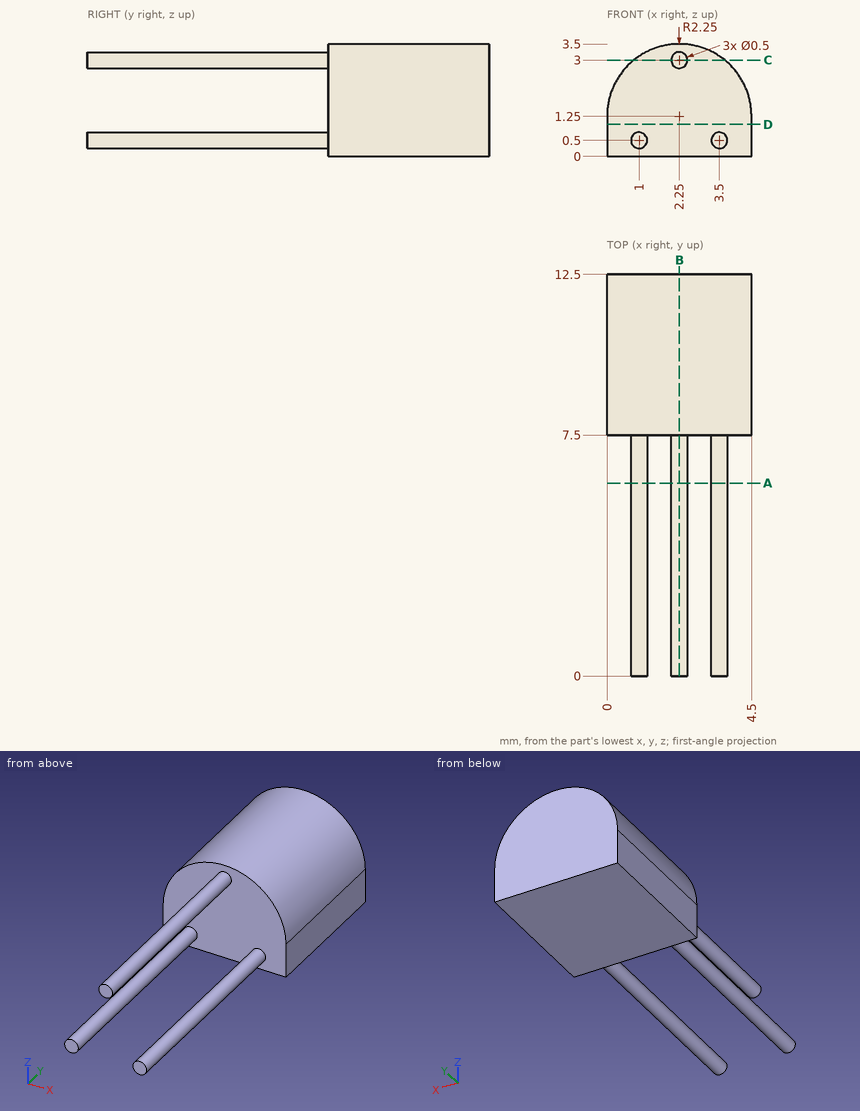
For this review, use the dimensioned drawing (mm, ordinates from the lowest corner) and the shaded views. Round coordinates to 2 decimals unless told otherwise and drop trailing zeros. Order: outer loops, then holes, each group sorted by start corner. A loop starts at its lowest first (then second) coordinate and runs counter-clockwise, first axis right, second up. Notation, with made-up numbers: M 89.25,-31 L 130.25,-31 A16 ccw 130.25,0 Z; hole C -30.75,75 d3. An arc over 180 degrees is marked long. Use a Markdown table: item, result.
1) Consider section D-D (z = 1). Write out the cut boundary in (x, y), then the cut area to 3 significant figures.
Report:
| item | result |
|---|---|
| outline | M 0,7.5 L 4.5,7.5 L 4.5,12.5 L 0,12.5 Z |
| area | 22.5 mm^2 |
2) Insertion check: pin 1 (1 mm diameter, centred on x = 2, z = 2.5, fed in from -Y). The pin has a flat end and moves straight along its axis. Give the tip position at first contact, or say it passes through.
Report:
| item | result |
|---|---|
| pin 1 | y = 0 |
3) Wall thickness on line 1 along Y through (x, z) = (0.8, 1.1); line 2 along X through (y, z) = (0.75, 0.35); line 3 along X through (y, z) = (9, 1.8): over which ranges is each line inside the solid? List them lowest first. Write a range as [from, to].
Report:
| item | result |
|---|---|
| line 1 | [7.5, 12.5] |
| line 2 | [0.8, 1.2], [3.3, 3.7] |
| line 3 | [0.07, 4.43] |
4) Consider section B-B (x = 2.25). Write out the cut boundary in (y, z), then the cut area to 4 significant figures.
Report:
| item | result |
|---|---|
| outline | M 0,2.75 L 7.5,2.75 L 7.5,0 L 12.5,0 L 12.5,3.5 L 7.5,3.5 L 7.5,3.25 L 0,3.25 Z |
| area | 21.25 mm^2 |
5) Consider section A-A (y = 6). Write out the cut boundary in (x, z).
Report:
| item | result |
|---|---|
| outline | C 1,0.5 d0.5; C 2.25,3 d0.5; C 3.5,0.5 d0.5 |
6) Consider section C-C (z = 3). Write out the cut boundary in (x, y), then the cut area to 3 significant figures.
Report:
| item | result |
|---|---|
| outline | M 0.84,7.5 L 2,7.5 L 2,0 L 2.5,0 L 2.5,7.5 L 3.66,7.5 L 3.66,12.5 L 0.84,12.5 Z |
| area | 17.9 mm^2 |
